Verification items for the finished model (mm, model axes). A direction names the side the tool comes from. Coordinates: 2 decimals unless noted, no trailing zeros. Order: outer loops, then holes, each group sorted by start corner. A loop starts at its lowest first (then second) coordinate and runs counter-clockwise, first axis right, second up. Notation, with made-up numbers: (29.5, 76) -> (40.5, 76) arc R21 ccw to (40.5, 104) -> close; hole circle Ø2 at (7, 59). An arc over 180 degrees is marked (long way). Write each question's results on one line, items separated by ' | '. Start each with the question number.
(1) Thickness scan on probe 1 along X at (y, z) = (1.5, 6.75); probe 2 along X at (y, z) = (3.5, -3.15); probe 3 along Z at (x, y) = (10.5, 5.5). Record the ranges inside material, lowest first. Write a range as [from, to].
(2) Set-up check for faces 4 (the flat face through (0, 2, 11)), 5 (the flat face through (-11, 4, 8)), 6 (the flat face through (-17, 2, 3)), 7 (the flat face through (-6, 0, 1)): record each of +Z, -Z, +X, -X, +Y, -Y from which the full face is reachable in a straight line by a thin tool's end or side.
(3) Cross-section at A-A on x = -11.75. Enter the section's corners in (y, z), and give its area (3 significant figures).
(4) Cross-section at C-C on z = -3.15. Enter the section's corners in (x, y), and give its area (3 significant figures).
(5) Cross-section at D-D on y = 2. Enter the section's corners in (x, z), and give its area (3 significant figures).
(6) Go/stop test with flat-tipped pins: pin 1 (2.5 mm diameter, centred on x = 11.75, z = 6.75, fed in from +Y); pin 2 (4 mm diameter, centred on y = 5.5, z = -2, fed in from -X); pin 3 (3 mm diameter, centred on x = -10.5, y = 2, fed in from -Z). Record where each tip stops, or that it passes through.
(7) Draft check along Z on faces 1 (the flat face through (-13, 2, 0.5)), 2 (the flat face through (2, 4, 2.5)), 3 (the flat face through (-6, 2, 13)). Enter one of: +Z half, -Z half, draft (parallel to the pull), parting line (faces both ways), or undercut.
(8) Cross-section at B-B on z = 3.5. Enter the section's corners in (x, y), and give its area (3 significant figures).
```python
from build123d import *

# Parameters (mm, degrees)
SZKIC1_R                    = 1
SZKIC1_W                    = 20.2
SZKIC1_H                    = 8.5
DODANIE_WYCI_GNI_CIE2_DEPTH = 4
SZKIC3_W                    = 13
SZKIC3_H                    = 9
DODANIE_WYCI_GNI_CIE3_DEPTH = 4
SZKIC1_3_R                  = 1
WYTNIJ_WYCI_GNI_CIE2_DEPTH  = 32.016124839
SZKIC4_R                    = 1
WYTNIJ_WYCI_GNI_CIE3_DEPTH  = 10


with BuildPart() as part:
    # Szkic1 → Dodanie-wyci_gni_cie2 (new body)
    with BuildSketch(Plane(origin=(0, 0, 0), x_dir=(1, 0, 0), z_dir=(0, 1, 0))):
        Polygon((-27, -0.5), (0.5, -0.5), (0.5, 6.5), (13.5, 6.5), (13.5, -13), (-27, -13), align=None)
        with Locations(Location((11.75, -6.75, 0), (0, 0, 270))):
            Circle(SZKIC1_R, mode=Mode.SUBTRACT)
        with Locations(Location((-11.75, -6.75, 0), (0, 0, 270))):
            Circle(SZKIC1_R, mode=Mode.SUBTRACT)
        with Locations(Location((3.5, 3.15, 0), (0, 0, 270))):
            Circle(SZKIC1_R, mode=Mode.SUBTRACT)
        with Locations(Location((10.5, 3.15, 0), (0, 0, 270))):
            Circle(SZKIC1_R, mode=Mode.SUBTRACT)
        with Locations((0, -6.75)):
            Rectangle(SZKIC1_W, SZKIC1_H, mode=Mode.SUBTRACT)
    extrude(amount=DODANIE_WYCI_GNI_CIE2_DEPTH)

    # Szkic3 → Dodanie-wyci_gni_cie3 (add)
    with BuildSketch(Plane.XZ.offset(-4)):
        with Locations((7, -2)):
            Rectangle(SZKIC3_W, SZKIC3_H)
    extrude(amount=-DODANIE_WYCI_GNI_CIE3_DEPTH)

    # Szkic1_3 → Wytnij-wyci_gni_cie2 (cut, through all)
    with BuildSketch(Plane(origin=(0, 0, 0), x_dir=(1, 0, 0), z_dir=(0, 1, 0))):
        with Locations(Location((10.5, 3.15, 0), (0, 0, 270))):
            Circle(SZKIC1_3_R)
        with Locations(Location((3.5, 3.15, 0), (0, 0, 270))):
            Circle(SZKIC1_3_R)
    extrude(amount=WYTNIJ_WYCI_GNI_CIE2_DEPTH, mode=Mode.SUBTRACT)

    # Szkic4 → Wytnij-wyci_gni_cie3 (cut)
    with BuildSketch(Plane.ZY.offset(27)):
        with Locations((3.5, 2)):
            Circle(SZKIC4_R)
        with Locations((10, 2)):
            Circle(SZKIC4_R)
    extrude(amount=-WYTNIJ_WYCI_GNI_CIE3_DEPTH, mode=Mode.SUBTRACT)


solid = part.part
```
Results are:
1) probe 1: x = [-27, -12.75], [-10.75, -10.1], [10.1, 10.75], [12.75, 13.5] | probe 2: x = [0.5, 2.5], [4.5, 9.5], [11.5, 13.5] | probe 3: z = [-6.5, -4.15], [-2.15, 2.5]
2) face 4: +Y, -Y | face 5: +Z, -X, +Y | face 6: -X | face 7: +Z, -Z, +X, -X, -Y
3) outline: (0, 0.5) -> (4, 0.5) -> (4, 5.75) -> (0, 5.75) -> close; (0, 7.75) -> (4, 7.75) -> (4, 13) -> (0, 13) -> close | area: 42.0 mm2
4) outline: (0.5, 0) -> (2.5, 0) -> (2.5, 8) -> (0.5, 8) -> close; (4.5, 0) -> (9.5, 0) -> (9.5, 8) -> (4.5, 8) -> close; (11.5, 0) -> (13.5, 0) -> (13.5, 8) -> (11.5, 8) -> close | area: 72.0 mm2
5) outline: (-27, 0.5) -> (0.5, 0.5) -> (0.5, -6.5) -> (13.5, -6.5) -> (13.5, 13) -> (-27, 13) -> (-27, 11) -> (-17, 11) -> (-17, 9) -> (-27, 9) -> (-27, 4.5) -> (-17, 4.5) -> (-17, 2.5) -> (-27, 2.5) -> close; hole circle Ø2 at (-11.75, 6.75); hole (-10.1, 2.5) -> (10.1, 2.5) -> (10.1, 11) -> (-10.1, 11) -> close; hole circle Ø2 at (3.5, -3.15); hole circle Ø2 at (10.5, -3.15); hole circle Ø2 at (11.75, 6.75) | area: 373 mm2
6) pin 1: stops at y = 4 | pin 2: stops at x = 0.5 | pin 3: stops at z = 0.5
7) face 1: -Z half | face 2: undercut | face 3: +Z half
8) outline: (-27, 0) -> (-10.1, 0) -> (-10.1, 4) -> (-27, 4) -> (-27, 3) -> (-17, 3) -> (-17, 1) -> (-27, 1) -> close; (10.1, 0) -> (13.5, 0) -> (13.5, 4) -> (10.1, 4) -> close | area: 61.2 mm2
